```python
from build123d import *

# Parameters (mm, degrees)
ESQUISSE1_R        = 7.66384886
BOSS_EXTRU_1_DEPTH = 2
CONG_1_R           = 10
CONG_2_R           = 1


# Some blends are built 0.0001 mm under size
with BuildPart() as part:
    # Esquisse1 → Boss.-Extru.1 (new body)
    with BuildSketch(Plane.XY):
        with BuildLine():
            Line((0, 0), (34, 0))
            Line((34, 0), (34, 22))
            Line((34, 22), (42, 22))
            Line((42, 22), (42, 0))
            ThreePointArc((42, 0), (17, -23.15919806), (-8, 0))
            Line((-8, 0), (-8, 22))
            Line((-8, 22), (0, 22))
            Line((0, 22), (0, 0))
        make_face()
        with Locations((17, -11.135898069)):
            Circle(ESQUISSE1_R, mode=Mode.SUBTRACT)
    extrude(amount=BOSS_EXTRU_1_DEPTH)

    # Congé1
    # the kernel refuses this fillet: 10 mm, written as the material it takes off along each edge
    with BuildSketch(Plane(origin=(42, 0, -1.388699458), x_dir=(0, 1, 0), z_dir=(0, 0, 1))) as cong_1_piece_1:
        with BuildLine():
            CenterArc((0.430691066, 10), CONG_1_R, 264.352690034, 5.647309966)
            ThreePointArc((-0.553355337, 0.048535149), (-0.276812081, 0.022735123), (0, 0))
            Line((0, 0), (0.430691066, 0))
        make_face()
    extrude(amount=4.777398915, mode=Mode.SUBTRACT)
    with BuildSketch(Plane(origin=(-8, 0, -1.388699458), x_dir=(0.08737518565273034, -0.9961754749702236, 0), z_dir=(0, 0, 1))) as cong_1_piece_2:
        with BuildLine():
            CenterArc((0.444707979, 9.999386462), CONG_1_R, 264.987378699, 5.647309966)
            Line((-0.429043877, 0.037631712), (0, 0))
            ThreePointArc((0, 0), (0.277739892, -0.001538335), (0.555479783, 0))
        make_face()
    extrude(amount=4.777398915, mode=Mode.SUBTRACT)

    # Congé2
    cong_2_edges = [part.edges().sort_by_distance(p)[0] for p in [
        (9.33615114, -11.135898069, 0),
        (9.33615114, -11.135898069, 2),
    ]]
    fillet(cong_2_edges, radius=CONG_2_R - 0.0001)  # a hair under: the kernel refuses the full size


solid = part.part
```
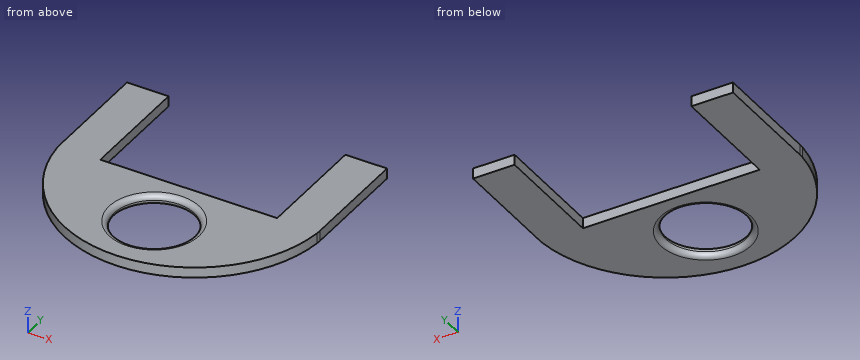
Source: CAD feature listing. Evaluate the final solid. Frame: model axes, mm. Coordinates: 2 decimals unless noted, no trailing zeros. Write each loop counter-clockwise with the first axis right and the second up, starting at its lowest first coordinate (ties: lowest second). Pieces come first, ordered by that corner, then holes. Notation, with made-up numbers: (45.5, -15.5) -> (76.5, -15.5) arc R24 ccw to (76.5, 18.5) -> close; hole circle Ø8 at (21, 46.5). An arc over 180 degrees is marked (long way). Return JSON: item names as keys, results as strings. Group by question number.
1) Section query C-C, the plane z = 1.45. Return loops of the section in (x, y), plus the area to 3 significant figures.
2) Section query B-B, the plane y = 16. Return loops of the section in (x, z).
3) Section query D-D, the plane x = 4. Return loops of the section in (y, z), plus the area to 3 significant figures.
4) Ray query, line 1 along Y through (x, z) = (17, 1); line 2 along X through (y, z) = (14.5, 0.65); line 3 along Y through (x, z) = (13.5, 0.7). Return the intervals inside material, ascending.
From the geometry:
{
 "1": {"outline": "(-8, 0.43) arc R10 ccw to (-7.95, -0.55) arc R25.07 ccw to (41.95, -0.55) arc R10 ccw to (42, 0.43) -> (42, 22) -> (34, 22) -> (34, 0) -> (0, 0) -> (0, 22) -> (-8, 22) -> close; hole circle Ø15.54 at (17, -11.14)", "area": "1,050 mm²"},
 "2": {"outline": "(-8, 0) -> (0, 0) -> (0, 2) -> (-8, 2) -> close; (34, 0) -> (42, 0) -> (42, 2) -> (34, 2) -> close"},
 "3": {"outline": "(-19.53, 0) -> (0, 0) -> (0, 2) -> (-19.53, 2) -> close", "area": "39.1 mm²"},
 "4": {"line 1": "-23.16 to -18.8, -3.47 to 0", "line 2": "-8 to 0, 34 to 42", "line 3": "-22.91 to -18.01, -4.27 to 0"}
}
